from build123d import *

# Parameters (mm, degrees)
ESQUISSE1_W       = 10
ESQUISSE1_H       = 5
EXTRUSION1_DEPTH  = 15
TROU_TARAUD_M31_D = 2.5
TROU_TARAUD_M32_D = 2.5
TROU_TARAUD_M33_D = 2.5


with BuildPart() as part:
    # Esquisse1 → Extrusion1 (new body)
    with BuildSketch(Plane.XY):
        with Locations((5, 2.5)):
            Rectangle(ESQUISSE1_W, ESQUISSE1_H)
    extrude(amount=EXTRUSION1_DEPTH)

    # Trou taraudé M31 (through all)
    with Locations(Plane.XY.offset(15)):
        with Locations((5, 2.5)):
            Hole(TROU_TARAUD_M31_D / 2)

    # Trou taraudé M32 (through all)
    with Locations(Plane(origin=(10, 0, 0), x_dir=(0, 0, -1), z_dir=(1, 0, 0))):
        with Locations((-7.5, 2.5)):
            Hole(TROU_TARAUD_M32_D / 2)

    # Trou taraudé M33 (through all)
    with Locations(Plane(origin=(0, 5, 0), x_dir=(-1, 0, 0), z_dir=(0, 1, 0))):
        with Locations((-5, 11.5), (-5, 3.5)):
            Hole(TROU_TARAUD_M33_D / 2)


solid = part.part
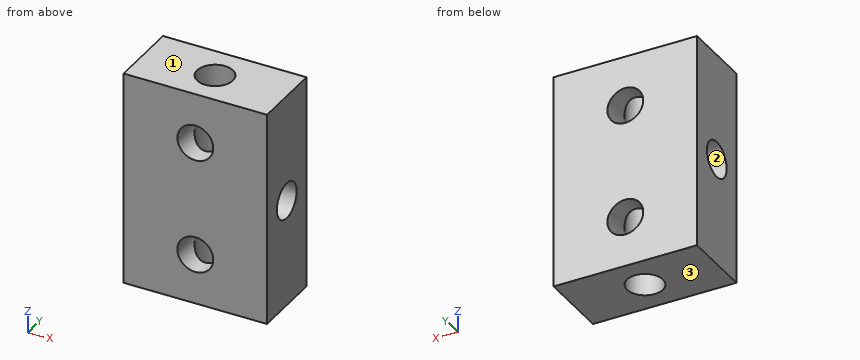
Check sheet for the modelled part. Datum: model origin and axes. Units: mm. Face numbers are marked on the shaded views. Give positions to 0.01 mm unless a question says otherwise; leave off trailing zeros. Write each loop counter-clockwise with the first axis right and the second up, starting at its lowest first coordinate (ties: lowest second). Pieces come first, ordered by that corner, then holes. Notation, with made-up numbers: M -13.75,24 L 15.25,24 A25 ccw 15.25,47 Z; hole C 82,16.5 d7. An arc over 180 degrees is marked long. Use one line per item in the form item = value.
(1) Section check D-D on z = 13. Record the boundary of the cut face in (x, y).
Answer block:
outline = M 0,0 L 10,0 L 10,5 L 0,5 Z; hole C 5,2.5 d2.5
(2) Section check C-C on y = 2.15. Record the boundary of the cut face in (x, z).
Answer block:
outline = M 0,0 L 3.8,0 L 3.8,3.15 A1.25 cw 3.8,3.85 L 3.8,6.3 L 0,6.3 Z; M 0,8.7 L 3.8,8.7 L 3.8,11.15 A1.25 cw 3.8,11.85 L 3.8,15 L 0,15 Z; M 6.2,0 L 10,0 L 10,6.3 L 6.2,6.3 L 6.2,3.85 A1.25 cw 6.2,3.15 Z; M 6.2,8.7 L 10,8.7 L 10,15 L 6.2,15 L 6.2,11.85 A1.25 cw 6.2,11.15 Z
(3) Section check A-A on z = 4.5. Record the boundary of the cut face in (x, y).
Answer block:
outline = M 0,0 L 4.25,0 L 4.25,1.5 A1.25 cw 4.25,3.5 L 4.25,5 L 0,5 Z; M 5.75,0 L 10,0 L 10,5 L 5.75,5 L 5.75,3.5 A1.25 cw 5.75,1.5 Z
(4) Section check B-B on x = 4. Record the boundary of the cut face in (y, z), plus the area to 3 significant figures.
Answer block:
outline = M 0,0 L 1.75,0 L 1.75,2.75 L 0,2.75 Z; M 0,4.25 L 1.75,4.25 L 1.75,6.5 A1.25 cw 1.75,8.5 L 1.75,10.75 L 0,10.75 Z; M 0,12.25 L 1.75,12.25 L 1.75,15 L 0,15 Z; M 3.25,0 L 5,0 L 5,2.75 L 3.25,2.75 Z; M 3.25,4.25 L 5,4.25 L 5,10.75 L 3.25,10.75 L 3.25,8.5 A1.25 cw 3.25,6.5 Z; M 3.25,12.25 L 5,12.25 L 5,15 L 3.25,15 Z
area = 40.6 mm2
(5) Depth check by flat-ended pin: P1, Ø2, axis at y = 2.5, z = 7.5, coming from the -X side. Enter the tip coordinate at first touch or a pass-through.
Answer block:
P1 = through
(6) Material ranges on line 1 along Z through (x, y) = (5, 0.9); line 2 along Y through (x, z) = (7.45, 7.5); line 3 along X through (y, z) = (2.5, 2.35), recorded low to high.
Answer block:
line_1 = 0 to 2.25, 4.75 to 10.25, 12.75 to 15
line_2 = 0 to 1.25, 3.75 to 5
line_3 = 0 to 3.75, 6.25 to 10
(7) Draft check along Z on the marked faces 1, 2 and 3. Enter one of: pulls with the +Z half, pulls with the -Z half, needs draft (parallel to the pull), parting line crosses it, or undercut.
Answer block:
face_1 = pulls with the +Z half
face_2 = undercut
face_3 = pulls with the -Z half
